The listing builds one solid part. Answer for the finished solid, in the listing's coordinates (mm). A direction names the side the tool comes from. Give positions to 0.01 mm unless a question says otherwise; leave off trailing zeros. Write each loop counter-clockwise with the first axis right and the second up, starting at its lowest first coordinate (ties: lowest second). Pieces come first, ordered by that corner, then holes.
Autodesk Inventor part; units mm, degrees
ref_plane "YZ Plane" through (0, 0, 0) normal (1, 0, 0) x (0, 1, 0)
ref_plane "XZ Plane" through (0, 0, 0) normal (0, 1, 0) x (-1, 0, 0)
ref_plane "XY Plane" through (0, 0, 0) normal (0, 0, 1) x (1, 0, 0)
sketch "Sketch1" plane through (0, 0, 0) normal (0, 1, 0) x (-1, 0, 0)
  line L0 (0, 0) -> (0, -1.3956)
  line L1 (1.5, 0) -> (2.8, 0)
  line L2 (2.8, 0) -> (2.8, -10)
  line L3 (2.8, -10) -> (2, -10)
  line L4 (2, -10) -> (2, -0.5)
  line L5 (2, -5.9601) -> (0.25, -5.9601)
  line L6 (0.25, -5.9601) -> (0.25, -5.5601)
  line L7 (0.25, -5.5601) -> (2, -3.8101)
  line L8 (2, -3.8101) -> (2, -5.9601)
  line L9 (2.8, -4.4) -> (-2.8, -10)
  line L10 (-2.8, -10) -> (2.8, -10)
  line L11 (-2.8, -10) -> (-2.0623, -10)
  line L12 (2, -0.5) -> (1.5, 0)
  line L13 (0, -7.2) -> (0, -7.7) construction
  line L14 (0, -7.7) -> (-4.7359, -7.7)
  line L15 (-4.7359, -7.7) -> (-4.7359, -2.9641)
  line L16 (-4.7359, -2.9641) -> (0, -7.7)
  point P0 (2, -3.8101)
  point P1 (0, -10)
  point P2 (2, -10)
  point P3 (2, -5.2)
  point P4 (0.9439, -6.2561)
  point P5 (1.2399, -5.9601)
  point P6 (0.2, -7)
  point P7 (2, -5.2)
  point P8 (-0.5, -7.7)
  point P9 (-0.25, -7.45)
  dimension "d1" = 10
  dimension "d4" = 2
  dimension "d10" = 45
  dimension "d19" = 0.8
  dimension "d21" = 1.5
  dimension "d23" = 45
  dimension "d24" = 45
  dimension "d25" = 0.25
  dimension "d26" = 0.4
  dimension "d27" = 0.7
  dimension "d30" = 0.5
  dimension "d31" = 45
revolve "Revolution1" add sketch "Sketch1" angle 360 about axis through (0, 0, 0) along (0, 0, -1) contours L1 L2 L9 L4 L12 | L2 L3 L4 L9 | L4 L9 L5 L6 L7 | L4 L5 L9
extrude "Extrusion4" cut sketch "Sketch1" along normal mid plane 25.4 contours L2 L3 L4 L9 | L4 L5 L9 | L10 L9 L14 L16 L5 L4 | L16 L14 L9
revolve "Revolution3" cut sketch "Sketch1" angle 360 about axis through (0, 0, -7.7) along (1, 0, 0) contours L9 L14 L15 L16
properties part number "aperature"
Item 1: A cutting plane is placed at D-D, the plane z = -3. Give the vertices of the cut face in (x, y), plus the area to 3 significant figures.
Conclusion:
outline: circle Ø5.6 at (0, 0); hole circle Ø4 at (0, 0)
area: 12.1 mm2
Item 2: Each of these flat-tipped pins is pushed along its axis until it touches: P1, Ø3, axis at y = -2, z = -5, coming from the +X side (3 decimals); P2, Ø2, axis at x = -0.5, y = 0.5, coming from the +Z side; P3, Ø0.9, axis at x = -0.5, y = 0.5, coming from the -Z side; P4, Ø1, axis at y = -1.5, z = -3, coming from the -X side. Where does it stop, or does it pass through?
Conclusion:
P1: stops at x = 2.755
P2: stops at z = 0
P3: stops at z = -5.96
P4: stops at x = -2.62
Item 3: Which of the six approach directions +Z, -Z, +X, -X, +Y, -Y give full straight-line access (tool end or side, diameter ignored) to faces 1 (the face through (2, 0.1, -5.7)), 2 (the face through (0.904, -1.784, -6.735)), 3 (the face through (0.44, 0.337, -5.256))?
Conclusion:
face 1: +X
face 2: -Z
face 3: none
Item 4: Determine the mould class of faces 4 (the face through (0, -2, 0)), 5 (the face through (2.8, 0.1, -2.7)), 6 (the face through (0.56, 1.92, -6.73)) for opening direction X: pulls with the +X half, pulls with the -X half, needs draft (parallel to the pull), parting line crosses it, or undercut.
Conclusion:
face 4: needs draft
face 5: parting line crosses it
face 6: undercut
Item 5: A cutting plane is placed at A-A, the plane x = 0. Give the vertices of the cut face in (y, z).
Conclusion:
outline: (-2.8, -7.2) - (-2, -7.2) - (-2, -5.96) - (-0.25, -5.96) - (-0.25, -5.56) - (-2, -3.81) - (-2, -0.5) - (-1.5, 0) - (-2.8, 0) - close; (0.25, -5.96) - (2, -5.96) - (2, -7.2) - (2.8, -7.2) - (2.8, 0) - (1.5, 0) - (2, -0.5) - (2, -3.81) - (0.25, -5.56) - close
Item 6: A cutting plane is placed at C-C, the plane z = -7.7. Give the vertices of the cut face in (x, y) (1 decimal).
Conclusion:
outline: (0.5, -2.8) arc R2.8 ccw to (2, -2) - (1.4, -1.4) arc R2 cw to (0.5, -1.9) - close; (0.5, 1.9) arc R2 cw to (1.4, 1.4) - (2, 2) arc R2.8 ccw to (0.5, 2.8) - close
Item 7: Consider probe 1 along Y at (x, z) = (0, -5.75); probe 2 along Y at (x, z) = (-1, -2.5); probe 3 along Z at (x, y) = (1.7, 1). Determine where each line is inside the solid, lowest interval first.
Conclusion:
probe 1: y = -2.8 to -0.25, 0.25 to 2.8
probe 2: y = -2.62 to -1.73, 1.73 to 2.62
probe 3: z = -5.96 to -3.84, -0.47 to 0
Item 8: A cutting plane is placed at B-B, the plane y = 0. Give the vertices of the cut face in (x, z).
Conclusion:
outline: (-2.8, -4.4) - (-1.24, -5.96) - (-0.25, -5.96) - (-0.25, -5.56) - (-2, -3.81) - (-2, -0.5) - (-1.5, 0) - (-2.8, 0) - close; (0.25, -5.96) - (1.74, -5.96) - (2.8, -4.9) - (2.8, 0) - (1.5, 0) - (2, -0.5) - (2, -3.81) - (0.25, -5.56) - close
